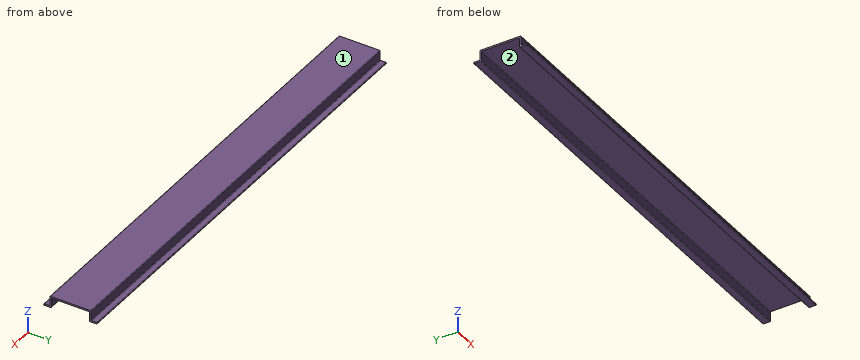
from build123d import *

# Parameters (mm, degrees)
SALIENTE_EXTRUIR1_DEPTH      = 150
SALIENTE_EXTRUIR1_DEPTH_BACK = 150
REDONDEO1_R                  = 0.5


with BuildPart() as part:
    # Croquis1 → Saliente-Extruir1 (new, two sides: drawn at the far end of the back side and taken through both)
    with BuildSketch(Plane(origin=(0, 0, 0), x_dir=(0, 0, -1), z_dir=(1, 0, 0)).offset(-SALIENTE_EXTRUIR1_DEPTH_BACK)):
        Polygon((0, 0), (0, 13.5), (6.5, 13.5), (6.5, 17.5), (7.5, 17.5), (7.5, 12.5), (1, 12.5), (1, -12.5), (7.5, -12.5), (7.5, -17.5), (6.5, -17.5), (6.5, -13.5), (0, -13.5), align=None)
    extrude(amount=SALIENTE_EXTRUIR1_DEPTH + SALIENTE_EXTRUIR1_DEPTH_BACK)

    # Redondeo1
    redondeo1_edges = [part.edges().sort_by_distance(p)[0] for p in [
        (0, 12.5, -1),
        (0, 12.5, -7.5),
        (0, 17.5, -7.5),
        (0, 17.5, -6.5),
        (0, 13.5, 0),
        (0, 13.5, -6.5),
        (0, -13.5, 0),
        (0, -13.5, -6.5),
        (0, -17.5, -6.5),
        (0, -17.5, -7.5),
        (0, -12.5, -7.5),
        (0, -12.5, -1),
    ]]
    fillet(redondeo1_edges, radius=REDONDEO1_R - 0.0001)  # a hair under: the kernel refuses the full size


solid = part.part
Input: part model. Units: mm. Frame: model coordinates. Face numbers are marked on the shaded views. A direction names the side the tool comes from. Coordinates: 2 decimals unless noted, no trailing zeros. Order: outer loops, then holes, each group sorted by start corner. A loop starts at its lowest first (then second) coordinate and runs counter-clockwise, first axis right, second up. Notation, with made-up numbers: M -12,20 L 39,20 A19 ccw 39,50 Z; hole C 24,89 d1. An arc over 180 degrees is marked long. One line per question, with ' | ' between items.
Item 1: Ray query, line 1 along Y through (x, z) = (107, -4); line 2 along Z through (x, y) = (-80, 4); line 3 along Y through (x, z) = (-71, -0.5). Return the intervals inside material, ascending.
Geometry results:
line 1: y = -13.5 to -12.5, 12.5 to 13.5 | line 2: z = -1 to 0 | line 3: y = -13.5 to 13.5
Item 2: Pin query (flat end, axial travel): pin 1 (1 mm diameter, centred on x = 11.5, z = -2, fed in from +Y); pin 2 (12 mm diameter, centred on x = 20, y = 1, fed in from -Z); pin 3 (2.5 mm diameter, centred on x = 36, y = 15, fed in from +Z); pin 4 (4 mm diameter, centred on y = 11, z = -3, fed in from +X). Return the tip coordinate at first contact, or that it passes through.
Geometry results:
pin 1: stops at y = 13.5 | pin 2: stops at z = -1 | pin 3: stops at z = -6.43 | pin 4: stops at x = 150
Item 3: Section C-C (y = -2). Output: boundary loops of the cut face in (x, z), then the cut area to 3 significant figures.
Geometry results:
outline: M -150,-1 L 150,-1 L 150,0 L -150,0 Z | area: 300 mm^2
Item 4: Section A-A (z = -3.5). Output: boundary loops of the cut face in (x, y), then the cut area to 3 significant figures.
Geometry results:
outline: M -150,-13.5 L 150,-13.5 L 150,-12.5 L -150,-12.5 Z; M -150,12.5 L 150,12.5 L 150,13.5 L -150,13.5 Z | area: 600 mm^2
Item 5: Reachability of the marked faces 1 and 2 from +Z, -Z, +X, -X, +Y, -Y: full face, straight path, thin tool, end or side. Return the list, or none.
Geometry results:
face 1: +Z, +X, -X, +Y, -Y | face 2: -Z, +X, -X
